The model under review builds one solid part; all positions refer to its coordinate system, in mm. Coordinates: 2 decimals unless noted, no trailing zeros. Loops run counter-clockwise (first coordinate to the right, second up) from the corner with the lowest first, then second, coordinate; pieces in that order, holes last. Notation, with made-up numbers: M 1.5,6 L 56.5,6 A18 ccw 56.5,26 Z; hole C 62,-24 d8. An arc over 180 degrees is marked long. Return JSON: item names as keys, results as strings.
Autodesk Inventor part; units mm, degrees
ref_plane "YZ Plane" through (0, 0, 0) normal (1, 0, 0) x (0, 1, 0)
ref_plane "XZ Plane" through (0, 0, 0) normal (0, 1, 0) x (-1, 0, 0)
ref_plane "XY Plane" through (0, 0, 0) normal (0, 0, 1) x (1, 0, 0)
sketch "Sketch1" plane through (0, 0, 0) normal (0, 1, 0) x (-1, 0, 0)
  line L0 (-19, -17) -> (19, -17)
  line L1 (19, -17) -> (19, 17)
  line L2 (19, 17) -> (-19, 17)
  line L3 (-19, 17) -> (-19, -17)
  line L4 (-19, -17) -> (19, 17) construction
  line L5 (19, -17) -> (-19, 17) construction
  point P0 (0, 0)
  dimension "d0" = 38
  dimension "d1" = 34
extrude "Extrusion1" add sketch "Sketch1" along normal blind 20
sketch "Sketch2" plane through (0, 0, 0) normal (0, -1, 0) x (1, 0, 0)
  arc A0 (0, 10) -> (0, -10) centre (0, 0) ccw
  line L0 (0, 10) -> (0, -23.7919) construction
  line L1 (0, -10) -> (0, 10)
  dimension "d4" = 20
revolve "Revolution1" cut sketch "Sketch2" angle 180 about axis through (0, 0, 10) along (0, 0, -1)
sketch "Sketch3" plane through (0, 0, 0) normal (0, -1, 0) x (1, 0, 0)
  point P0 (0, 0)
  point P1 (16, 12)
  point P2 (16, -12)
  point P3 (-16, -12.4929)
  point P4 (-16, 12)
hole "Hole1" at (-16, 0, -12.4929) at (-16, 0, 12) at (16, 0, 12) at (16, 0, -12) direction (0, 1, 0) diameter 3 end through all
properties part number "Box"
1. The part is to be moulded in two halves that separate along Z. For faces 1 (the face through (0, 10, 17)), 2 (the face through (-19, 10, 0)), 3 (the face through (-16.07, 10.14, 13.5)), say which applies: released by +Z, released by -Z, zero draft, split by the parting line, or undercut.
Check values:
{"face 1": "released by +Z", "face 2": "zero draft", "face 3": "undercut"}
2. Add section B-B on y = 16.5. Give the boundary of the cut face in (x, z), plus the area to 3 significant figures.
Check values:
{"outline": "M -19,-17 L 19,-17 L 19,17 L -19,17 Z; hole C -16,-12.49 d3; hole C -16,12 d3; hole C 16,-12 d3; hole C 16,12 d3", "area": "1,260 mm²"}
3. To check wall thickness, follow line 1 (X direction, y = 10.25, z = 12); line 2 (Z direction, x = 16, y = 9.5); line 3 (Z direction, x = -16, y = 8.5). State the ranges of each line that lie inside material, in increasing order.
Check values:
{"line 1": "-19 to -17.5, -14.5 to 14.5, 17.5 to 19", "line 2": "-17 to -13.5, -10.5 to 10.5, 13.5 to 17", "line 3": "-17 to -13.99, -10.99 to 10.5, 13.5 to 17"}
4. Add section A-A on x = 16. Give the boundary of the cut face in (y, z), plus the area to 3 significant figures.
Check values:
{"outline": "M 0,-17 L 20,-17 L 20,-13.5 L 0,-13.5 Z; M 0,-10.5 L 20,-10.5 L 20,10.5 L 0,10.5 Z; M 0,13.5 L 20,13.5 L 20,17 L 0,17 Z", "area": "560 mm²"}
5. Add section D-D on y = 1.5. Give the boundary of the cut face in (x, z), plus the area to 3 significant figures.
Check values:
{"outline": "M -19,-17 L 19,-17 L 19,17 L -19,17 Z; hole C -16,-12.49 d3; hole C -16,12 d3; hole C 0,0 d19.77; hole C 16,-12 d3; hole C 16,12 d3", "area": "957 mm²"}
6. Insertion check: pin 1 Ø2.5 at (x, z) = (-16, -12.49) entering from -Y. The pin has a flat end and moves straight along its axis. Give the tip position at first contact, or say it passes through.
Check values:
{"pin 1": "through"}
7. Add section C-C on z = 12. Give the boundary of the cut face in (x, y), plus the area to 3 significant figures.
Check values:
{"outline": "M -19,0 L -17.5,0 L -17.5,20 L -19,20 Z; M -14.5,0 L 14.5,0 L 14.5,20 L -14.5,20 Z; M 17.5,0 L 19,0 L 19,20 L 17.5,20 Z", "area": "640 mm²"}
